CAD build for the part. Positions are in the model's coordinates, mm. Face numbers are marked on the shaded views. A direction names the side the tool comes from. Give positions to 0.01 mm unless a question says otherwise; leave off trailing zeros. Write each loop counter-clockwise with the first axis right and the second up, starting at its lowest first coordinate (ties: lowest second). Pieces come first, ordered by that corner, then holes. Notation, with made-up numbers: (50.5, 23) -> (79.5, 23) arc R21 ccw to (79.5, 45) -> close; hole circle Ø6 at (-32, 5). An arc over 180 degrees is marked (long way). Answer in a Markdown table with one row per item. Add a question column.
```python
from build123d import *

# Parameters (mm, degrees)
SKETCH1_W               = 101.237370502
SKETCH1_H               = 95.893480298
BOSS_EXTRUDE1_DEPTH     = 5.08
CUT_EXTRUDE1_DEPTH      = 50.8
SKETCH3_W               = 34.377834067
SKETCH3_H               = 141.590062345
CUT_EXTRUDE2_DEPTH      = 25.4
SKETCH4_R               = 1.4224
CUT_EXTRUDE3_DEPTH      = 5.08
BOSS_EXTRUDE2_DEPTH     = 164.338
CUT_EXTRUDE4_DEPTH      = 152.4
CUT_EXTRUDE5_DEPTH      = 152.4
CUT_EXTRUDE5_DEPTH_BACK = 152.4
SKETCH8_W               = 19.066411764
SKETCH8_H               = 17.374579431
SKETCH8_W_2             = 17.073824451
CUT_EXTRUDE6_DEPTH      = 5.08


with BuildPart() as part:
    # Sketch1 → Boss-Extrude1 (new body)
    with BuildSketch(Plane.XY):
        with Locations((-50.618685251, 168.596740149)):
            Rectangle(SKETCH1_W, SKETCH1_H)
        Polygon((-101.237370502, 120.65), (0, 120.65), (0, 0), align=None)
    extrude(amount=BOSS_EXTRUDE1_DEPTH)

    # Sketch2 → Cut-Extrude1 (cut)
    with BuildSketch(Plane.XY.offset(5.08)):
        Polygon((-101.237370502, 216.543480298), (0, 108.271740149), (0, 216.543480298), align=None)
    extrude(amount=-CUT_EXTRUDE1_DEPTH, mode=Mode.SUBTRACT)

    # Sketch3 → Cut-Extrude2 (cut)
    with BuildSketch(Plane.XY.offset(5.08)):
        with Locations((5.61014441, 62.39317364)):
            Rectangle(SKETCH3_W, SKETCH3_H)
    extrude(amount=-CUT_EXTRUDE2_DEPTH, mode=Mode.SUBTRACT)

    # Sketch4 → Cut-Extrude3 (cut)
    with BuildSketch(Plane(origin=(0, 0, 0), x_dir=(0, 0, 1), z_dir=(-0.7660444431189743, -0.6427876096865437, 0))):
        with Locations(Location((2.54, 26.412934343, 0), (0, 0, 270))):
            Circle(SKETCH4_R)
        with Locations(Location((2.54, 153.412934343, 0), (0, 0, 270))):
            Circle(SKETCH4_R)
    extrude(amount=-CUT_EXTRUDE3_DEPTH, mode=Mode.SUBTRACT)

    # Sketch5 → Boss-Extrude2 (add)
    with BuildSketch(Plane.XY.offset(5.08)):
        Polygon((-101.237370502, 216.543480298), (-101.237370502, 221.697031777), (-43.160539618, 159.601331401), (15.407326332, 159.601331401), (15.407326332, 155.702260244), (-44.348979053, 155.702260244), align=None)
    extrude(amount=-BOSS_EXTRUDE2_DEPTH)

    # Sketch6 → Cut-Extrude4 (cut)
    with BuildSketch(Plane(origin=(0, 0, -63.5), x_dir=(-1, 0, 0), z_dir=(0, 0, -1))):
        Polygon((11.578772624, 120.655051318), (11.578772624, 13.799043873), (101.237370502, 120.65), (101.237370502, 216.543480298), align=None)
    extrude(amount=-CUT_EXTRUDE4_DEPTH, mode=Mode.SUBTRACT)

    # Sketch7 → Cut-Extrude5 (cut, two sides: drawn at the far end of the back side and taken through both)
    with BuildSketch(Plane(origin=(56.600313361, 52.937108481, 0), x_dir=(0, 0, -1), z_dir=(0.7303459019409237, 0.6830774945188128, 0)).offset(-CUT_EXTRUDE5_DEPTH_BACK)):
        Polygon((-5.08, 231.068488025), (7.526341611, 106.039780465), (-5.08, 106.039780465), align=None)
        Polygon((159.258, 231.068488025), (148.255408438, 106.039780465), (159.258, 106.039780465), align=None)
    extrude(amount=CUT_EXTRUDE5_DEPTH + CUT_EXTRUDE5_DEPTH_BACK, mode=Mode.SUBTRACT)

    # Sketch8 → Cut-Extrude6 (cut)
    with BuildSketch(Plane(origin=(15.407326332, 0, 0), x_dir=(0, 0, -1), z_dir=(1, 0, 0))):
        with Locations((-1.754260648, 156.68928868)):
            Rectangle(SKETCH8_W, SKETCH8_H)
        with Locations((156.594427777, 156.68928868)):
            Rectangle(SKETCH8_W_2, SKETCH8_H)
    extrude(amount=-CUT_EXTRUDE6_DEPTH, mode=Mode.SUBTRACT)


solid = part.part
```
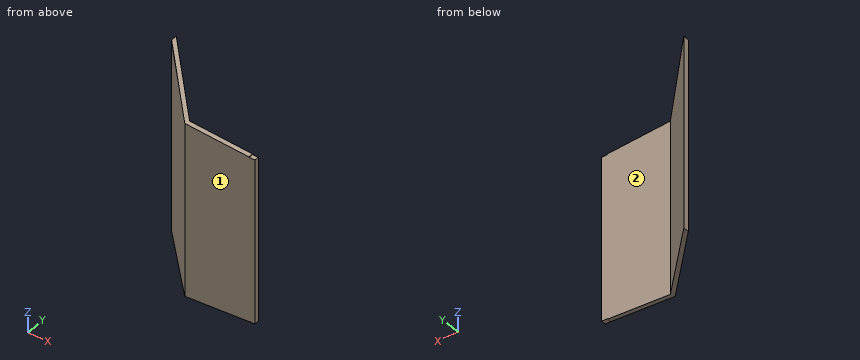
Item 1: Slice it at B-B, the plane x = -3.5. List the corners of the cut face in (y, z).
Item 2: Probe L1, parallel to Y at x = -40.5, z = -128.5; L2, parallel to X at y = 178, z = -37.5; L3, parallel to X at y = 185.5, z = -2.5. List the from-to ranges inside material, lowest first. Write a range as from..to.
Item 3: Slice it at C-C, the plane y = 191. List the corners of the cut face in (x, z), then the cut area to 3 significant figures.
Item 4: Drop flat-ended pins along their axis: pin 1 Ø3 at (x, y) = (14, 157.5) entering from +Z; pin 2 Ø8 at (x, y) = (-47.5, 168) entering from -Z; pin 3 Ø2 at (x, z) = (-53, -83) entering from +Y. Give the stop position or say it passes through.
Item 5: Which spindle directions (+Z, -Z, +X, -X, +Y, -Y) get a long thin tool onto all of the face, cutting with end or side? Do the marked faces 1 and 2. Say none if no direction does.
Item 6: Slice it at A-A, the plane z = -29.5. List the corners of the cut face in (x, y).
Answer key:
| question | item | result |
|---|---|---|
| 1 | outline | (155.7, -149.14) -> (159.6, -149.39) -> (159.6, -6.22) -> (155.7, -6.51) -> close |
| 2 | L1 | y = 155.7..159.6 |
| 2 | L2 | x = -65.2..-60.37 |
| 2 | L3 | x = -72.21..-67.38 |
| 3 | outline | (-77.35, -155.85) -> (-72.53, -155.56) -> (-72.53, 0.84) -> (-77.35, 1.17) -> close |
| 3 | area | 756 mm² |
| 4 | pin 1 | stops at z = -7.78 |
| 4 | pin 2 | stops at z = -152.85 |
| 4 | pin 3 | stops at y = 171.19 |
| 5 | face 1 | +Z, -Z, +X, -X, -Y |
| 5 | face 2 | +Z, -Z, +X, +Y |
| 6 | outline | (-101.24, 216.54) -> (-44.35, 155.7) -> (15.41, 155.7) -> (15.41, 159.6) -> (-43.16, 159.6) -> (-101.24, 221.7) -> close |
